```python
from build123d import *

# Parameters (mm, degrees)
F1_DEPTH = 3.81
F2_R     = 1.5748
F4_W     = 3.7084
F4_H     = 2.870018
F5_DEPTH = 0.7112


with BuildPart() as f1:
    # F0 (on Front) → F1 (new body)
    with BuildSketch(Plane.XZ):
        with BuildLine():
            ThreePointArc((-1.8542, 3.328369), (-1.930233, -3.284859), (3.81, 0))
            ThreePointArc((3.81, 0), (3.284859, 1.930233), (1.8542, 3.328369))
            ThreePointArc((1.8542, 3.328369), (0.957866, 3.687627), (0, 3.81))
            ThreePointArc((0, 3.81), (-0.957866, 3.687627), (-1.8542, 3.328369))
        make_face()
        with BuildLine():
            ThreePointArc((0, 3.81), (0.957866, 3.687627), (1.8542, 3.328369))
            Line((1.8542, 3.328369), (1.8542, 5.08))
            Line((1.8542, 5.08), (0, 5.08))
            Line((0, 5.08), (0, 3.81))
        make_face()
        with BuildLine():
            Line((-1.8542, 5.08), (-1.8542, 3.328369))
            ThreePointArc((-1.8542, 3.328369), (-0.957866, 3.687627), (0, 3.81))
            Line((0, 3.81), (0, 5.08))
            Line((0, 5.08), (-1.8542, 5.08))
        make_face()
    extrude(amount=-F1_DEPTH)

    # F2
    f2_edges = [f1.edges().sort_by_distance(p)[0] for p in [
        (1.8542, 1.905, 3.328369),
        (-1.8542, 1.905, 3.328369),
    ]]
    fillet(f2_edges, radius=F2_R)

    # F4 (on face) → F5 (cut)
    with BuildSketch(Plane.XY.offset(5.08)):
        with Locations((0, 1.435009)):
            Rectangle(F4_W, F4_H)
    extrude(amount=-F5_DEPTH, mode=Mode.SUBTRACT)


solid = f1.part
```
The listing builds one solid part. Answer for the finished solid, in the listing's coordinates (mm). A direction names the side the tool comes from. Round coordinates to 2 decimals unless told otherwise and drop trailing zeros. Write each loop counter-clockwise with the first axis right and the second up, starting at its lowest first coordinate (ties: lowest second). Pieces come first, ordered by that corner, then holes. Notation, with made-up numbers: (78, 76.5) -> (117, 76.5) arc R9 cw to (117, 82.5) -> close; hole circle Ø10 at (79, -22.75). An arc over 180 degrees is marked (long way). Answer as a JSON object with one key per item and string values. Group by question number.
Q1. Each of these flat-tipped pins is pushed along its axis until it touches: pin 1 Ø1 at (y, z) = (2.5, -2.5) entering from -X; pin 2 Ø1.4 at (x, y) = (0, 1) entering from +Z; pin 3 Ø0.5 at (y, z) = (2.5, 4.5) entering from +X. Where does it stop, or does it pass through?
Q2. Section D-D (x = 1.5) is taken. Write down the section's boundary in (y, z).
Q3. Section B-B (x = 0) is taken. Write down the section's boundary in (y, z), plus the area to 3 significant figures.
Q4. Which of the six approach directions +Z, -Z, +X, -X, +Y, -Y give full straight-line access (tool end or side, diameter ignored) to faces 1 (the face through (0, 1, 4.369)), 2 (the face through (1.854, 3.1, 4.4)), 3 (the face through (-1.854, 3.1, 4.4))?
Q5. Section C-C (z = 4.75) is taken. Write down the section's boundary in (x, y).
Q6. Section A-A (y = 1.4) is taken. Write down the section's boundary in (x, z).
Q7. Determine the mould class of faces 4 (the face through (2.01, 1.93, 3.47)), 5 (the face through (0, 3.81, 1)), 6 (the face through (0, 0, 0)) for opening direction Y: pulls with the +Y half, pulls with the -Y half, needs draft (parallel to the pull), parting line crosses it, or undercut.
Q8. Straight lines are drawn through the part: line 1 along Z through (x, y) = (-1.5, 0.25); line 2 along X through (y, z) = (2.2, -0.5); line 3 along Z through (x, y) = (-2.75, 2.15). For each, find the intervals that lie inside material, in ascending order.
Check values:
{
 "1": {"pin 1": "x = -3.24", "pin 2": "z = 4.37", "pin 3": "x = 1.85"},
 "2": {"outline": "(0, -3.5) -> (3.81, -3.5) -> (3.81, 5.08) -> (2.87, 5.08) -> (2.87, 4.37) -> (0, 4.37) -> close"},
 "3": {"outline": "(0, -3.81) -> (3.81, -3.81) -> (3.81, 5.08) -> (2.87, 5.08) -> (2.87, 4.37) -> (0, 4.37) -> close", "area": "31.8 mm^2"},
 "4": {"face 1": "+Z, +X, -X, -Y", "face 2": "+Z, +X, +Y, -Y", "face 3": "+Z, -X, +Y, -Y"},
 "5": {"outline": "(-1.85, 2.87) -> (1.85, 2.87) -> (1.85, 3.81) -> (-1.85, 3.81) -> close"},
 "6": {"outline": "(-2.43, 2.94) arc R3.81 ccw (long way) to (2.43, 2.94) arc R1.57 cw to (1.85, 4.15) -> (1.85, 4.37) -> (-1.85, 4.37) -> (-1.85, 4.15) arc R1.57 cw to start"},
 "7": {"face 4": "needs draft", "face 5": "pulls with the +Y half", "face 6": "pulls with the -Y half"},
 "8": {"line 1": "-3.5 to 4.37", "line 2": "-3.78 to 3.78", "line 3": "-2.64 to 2.64"}
}
